```python
from build123d import *

# Parameters (mm, degrees)
CYLINDER1977_R               = 3
CYLINDER1977_DEPTH           = 3
CYLINDER1974_R               = 3
CYLINDER1974_DEPTH           = 3
CYLINDER1975_R               = 3
CYLINDER1975_DEPTH           = 3
CYLINDER1976_R               = 3
CYLINDER1976_DEPTH           = 3
COMPOUND1064_PLACEMENT_ANGLE = 225
CYLINDER1981_R               = 1.5
CYLINDER1981_DEPTH           = 60
CYLINDER1978_R               = 1.5
CYLINDER1978_DEPTH           = 60
CYLINDER1979_R               = 1.5
CYLINDER1979_DEPTH           = 60
CYLINDER1980_R               = 1.5
CYLINDER1980_DEPTH           = 60
COMPOUND1067_PLACEMENT_ANGLE = 225
CYLINDER1982_R               = 74
CYLINDER1982_DEPTH           = 40
BOX982_W                     = 42
BOX982_H                     = 62
BOX982_DEPTH                 = 50
COMPOUND1065_PLACEMENT_ANGLE = 225
BOX983_W                     = 54
BOX983_H                     = 68
BOX983_DEPTH                 = 10
COMPOUND1066_PLACEMENT_ANGLE = 225
CHAMFER073_SIZE              = 3
CHAMFER074_SIZE              = 2
CHAMFER075_SIZE              = 1


with BuildPart() as obj1:
    # Cylinder1977 → Cylinder1977 (new body)
    with BuildSketch(Plane(origin=(-24, 74, -80), x_dir=(1, 0, 0), z_dir=(0, 0, 1))):
        Circle(CYLINDER1977_R)
    extrude(amount=CYLINDER1977_DEPTH)


with BuildPart() as obj2:
    # Cylinder1974 → Cylinder1974 (new body)
    with BuildSketch(Plane(origin=(-15, 135, -80), x_dir=(1, 0, 0), z_dir=(0, 0, 1))):
        Circle(CYLINDER1974_R)
    extrude(amount=CYLINDER1974_DEPTH)


with BuildPart() as obj3:
    # Cylinder1975 → Cylinder1975 (new body)
    with BuildSketch(Plane(origin=(15, 135, -80), x_dir=(1, 0, 0), z_dir=(0, 0, 1))):
        Circle(CYLINDER1975_R)
    extrude(amount=CYLINDER1975_DEPTH)


with BuildPart() as compound1064:
    # Cylinder1976 → Cylinder1976 (new body)
    with BuildSketch(Plane(origin=(24, 74, -80), x_dir=(1, 0, 0), z_dir=(0, 0, 1))):
        Circle(CYLINDER1976_R)
    extrude(amount=CYLINDER1976_DEPTH)

    # Compound1064: union obj1, obj2, obj3
    add(obj1.part)
    add(obj2.part)
    add(obj3.part)


with BuildPart() as compound1064_1:
    # Compound1064 placement: moved
    add(compound1064.part.moved(Location((0, 0, 135))).rotate(Axis((0, 0, 135), (0, 0, 1)), COMPOUND1064_PLACEMENT_ANGLE))


with BuildPart() as obj4:
    # Cylinder1981 → Cylinder1981 (new body)
    with BuildSketch(Plane(origin=(-24, 74, -80), x_dir=(1, 0, 0), z_dir=(0, 0, 1))):
        Circle(CYLINDER1981_R)
    extrude(amount=CYLINDER1981_DEPTH)


with BuildPart() as obj5:
    # Cylinder1978 → Cylinder1978 (new body)
    with BuildSketch(Plane(origin=(-15, 135, -80), x_dir=(1, 0, 0), z_dir=(0, 0, 1))):
        Circle(CYLINDER1978_R)
    extrude(amount=CYLINDER1978_DEPTH)


with BuildPart() as obj6:
    # Cylinder1979 → Cylinder1979 (new body)
    with BuildSketch(Plane(origin=(15, 135, -80), x_dir=(1, 0, 0), z_dir=(0, 0, 1))):
        Circle(CYLINDER1979_R)
    extrude(amount=CYLINDER1979_DEPTH)


with BuildPart() as compound1067:
    # Cylinder1980 → Cylinder1980 (new body)
    with BuildSketch(Plane(origin=(24, 74, -80), x_dir=(1, 0, 0), z_dir=(0, 0, 1))):
        Circle(CYLINDER1980_R)
    extrude(amount=CYLINDER1980_DEPTH)

    # Compound1067: union obj4, obj5, obj6
    add(obj4.part)
    add(obj5.part)
    add(obj6.part)


with BuildPart() as compound1067_1:
    # Compound1067 placement: moved
    add(compound1067.part.moved(Location((0, 0, 100))).rotate(Axis((0, 0, 100), (0, 0, 1)), COMPOUND1067_PLACEMENT_ANGLE))


with BuildPart() as obj7:
    # Cylinder1982 → Cylinder1982 (new body)
    with BuildSketch(Plane.XY.offset(44)):
        Circle(CYLINDER1982_R)
    extrude(amount=CYLINDER1982_DEPTH)


with BuildPart() as compound1065:
    # Box982 → Box982 (new body)
    with BuildSketch(Plane(origin=(-21.001071, 60.005081, 31), x_dir=(1, 0, 0), z_dir=(0, 0, 1))):
        with Locations((21, 31)):
            Rectangle(BOX982_W, BOX982_H)
    extrude(amount=BOX982_DEPTH)


with BuildPart() as compound1065_1:
    # Compound1065 placement: moved
    add(compound1065.part.rotate(Axis((0, 0, 0), (0, 0, 1)), COMPOUND1065_PLACEMENT_ANGLE))


with BuildPart() as cut664:
    # Box983 → Box983 (new body)
    with BuildSketch(Plane(origin=(-27.004408, 59.99801, 75), x_dir=(1, 0, 0), z_dir=(0, 0, 1))):
        with Locations((27, 34)):
            Rectangle(BOX983_W, BOX983_H)
    extrude(amount=BOX983_DEPTH)


with BuildPart() as cut664_1:
    # Compound1066 placement: moved
    add(cut664.part.moved(Location((0, 0, -20))).rotate(Axis((0, 0, -20), (0, 0, 1)), COMPOUND1066_PLACEMENT_ANGLE))

    # Cut666: cut Compound1065
    add(compound1065_1.part, mode=Mode.SUBTRACT)

    # Cut669: cut obj7
    add(obj7.part, mode=Mode.SUBTRACT)

    # Chamfer073
    chamfer073_edges = [cut664_1.edges().sort_by_distance(p)[0] for p in [
        (109.603261, -71.413261, 60),
        (71.419495, -109.597027, 60),
    ]]
    chamfer(chamfer073_edges, length=CHAMFER073_SIZE)

    # Chamfer074
    chamfer074_edges = [cut664_1.edges().sort_by_distance(p)[0] for p in [
        (87.647149, -49.457149, 55),
        (49.464605, -87.642137, 55),
    ]]
    chamfer(chamfer074_edges, length=CHAMFER074_SIZE)

    # Chamfer075
    chamfer075_edges = [cut664_1.edges().sort_by_distance(p)[0] for p in [
        (90.511378, -90.505144, 55),
    ]]
    chamfer(chamfer075_edges, length=CHAMFER075_SIZE)

    # Cut665: cut Compound1067
    add(compound1067_1.part, mode=Mode.SUBTRACT)

    # Cut664: cut Compound1064
    add(compound1064_1.part, mode=Mode.SUBTRACT)


solid = cut664_1.part
```
CAD build for the part. Positions are in the model's coordinates, mm. A direction names the side the tool comes from. Round coordinates to 2 decimals unless told otherwise and drop trailing zeros. Order: outer loops, then holes, each group sorted by start corner. A loop starts at its lowest first (then second) coordinate and runs counter-clockwise, first axis right, second up.
Q1. Slice it at D-D (x = 44). Write the cut outline in (y, z), and give its area (3 significant figures).
Q2. Two-plate mould, pull along Y, no slides. Class faces 4 (the cylindrical face through (35.782, -66.327, 56.479)), 5 (the flat face through (36, -71, 58)), 6 (the flat face through (52.47, -89.25, 56.01)), 7 (the flat face through (66, -34, 55)): pulls with the +Y half, pulls with the -Y half, needs draft (parallel to the pull), parting line crosses it, or undercut.
Q3. Which spindle directions (+Z, -Z, +X, -X, +Y, -Y) get a long thin tool onto all of the face, cutting with end or side? Do faces 1 (the flat face through (31.5, -68.6, 56.24)), 2 (the flat face through (53.122, -82.819, 59.93)), 3 (the flat face through (70, -37, 58)). Say none if no direction does.
Q4. Slice it at B-B (x = 93). Write the cut outline in (y, z).
Q5. Drop flat-ended pins along their axis: pin 1 (3 mm diameter, centred on y = -76.5, z = 57.5, fed in from -X); pin 2 (5 mm diameter, centred on x = 70.5, y = -35, fed in from -Z); pin 3 (3 mm diameter, centred on x = 34.5, y = -70, fed in from -Z); pin 4 (3 mm diameter, centred on x = 88.5, z = 60.5, fed in from +Y). Give the stop position or say it passes through.
Q6. Wall check: L1, parallel to Y at x = 100, z = 62; L2, parallel to X at y = -76, z = 55.75; L3, parallel to Y at x = 87, z = 59. Give the ranges that are in metal, low to high.
Q7. Slice it at C-C (z = 63.5). Write the cut outline in (x, y).
Q8. Slice it at A-A (y = -94). Write the cut outline in (x, z), and give its area (3 significant figures).
Results below:
1. outline: (-82.18, 57) - (-79.35, 55) - (-73.7, 55) - (-73.7, 65) - (-82.18, 65) - close
1. area: 82.0 mm2
2. face 4: undercut
2. face 5: undercut
2. face 6: pulls with the -Y half
2. face 7: needs draft
3. face 1: -Z, -X, -Y
3. face 2: +Z, -Z
3. face 3: -Z
4. outline: (-88.02, 56) - (-86.6, 55) - (-79.54, 55) - (-79.54, 65) - (-88.02, 65) - close; (-63.3, 55) - (-57.64, 55) - (-54.81, 57) - (-54.81, 65) - (-63.3, 65) - close
5. pin 1: stops at x = 36.82
5. pin 2: stops at z = 55
5. pin 3: stops at z = 58
5. pin 4: stops at y = -48.81
6. L1: y = -81.02 to -72.54, -70.3 to -61.81
6. L2: x = 39.59 to 46.3, 96.54 to 104.66
6. L3: y = -94.02 to -85.54, -57.3 to -48.81
7. outline: (29.63, -67.81) - (69.3, -107.48) - (73.54, -107.48) - (107.48, -73.53) - (107.48, -69.29) - (67.81, -29.62) arc R74 cw to (65.02, -35.32) - (101.12, -71.42) - (71.42, -101.12) - (35.33, -65.02) arc R74 cw to start; hole circle Ø3 at (35.36, -69.3); hole circle Ø3 at (69.3, -35.36)
8. outline: (55.82, 57) - (58.65, 55) - (64.3, 55) - (64.3, 65) - (55.82, 65) - close; (78.54, 55) - (85.6, 55) - (87.02, 56) - (87.02, 65) - (78.54, 65) - close
8. area: 166 mm2
